Read the model definition and answer for the solid it produces. Units are mm, in the model's axes. A direction names the side the tool comes from. Give positions to 0.01 mm unless a question says otherwise; leave off trailing zeros. Write each loop counter-clockwise with the first axis right and the second up, starting at its lowest first coordinate (ties: lowest second). Pieces come first, ordered by that corner, then holes. Notation, with made-up numbers: M -15.5,-13.75 L 6.5,-13.75 A14 ccw 6.5,-3.75 Z; hole C 4,89 d8. An arc over 180 degrees is marked long. Use a Markdown table: item, result. Add a question column.
Item 1: Consider probe 1 along Y at (x, z) = (-22.5, -4.05); probe 2 along Y at (x, z) = (-52.5, -2.9); probe 3 along X at (y, z) = (-2, -3.85). Determine where each line is inside the solid, lowest interval first. Write a range as [from, to].
Item 2: A cutting plane is placed at A-A on z = -3.55. Determine the outline of the cut face in (x, y), then the cut area to 3 significant figures.
Item 3: The mould has two halves that part along X. Classify faces 1 (the flat face through (-36.032, -10.535, -2.958)), 2 (the flat face through (-38.34, 4.12, -2.96)), 3 (the flat face through (-37.19, -9.23, -2.96)): pulls with the +X half, pulls with the -X half, needs draft (parallel to the pull), parting line crosses it, or undercut.
Item 4: Given P1, Ø1, axis at x = -25.5, y = 4.5, coming from the +Z side; P2, Ø2, axis at y = -9.5, z = -2, coming from the -X side; P3, Ø1, axis at y = -6.5, z = -4.5, coming from the +X side; P4, Ø1, axis at y = -5.5, z = -1.5, coming from the -X side, each flat-ended and moving along its own axis, determine where each tip first touches the part or whether it passes through.
Item 5: A cutting plane is placed at C-C on x = -33.5. Determine the outline of the cut face in (y, z), then the cut area to 3 significant figures.
Item 6: For faces 4 (the flat face through (-37.183, 2.815, -2.958)), 5 (the flat face through (-37.4, -9.4, -6)), determine the directions among +Z, -Z, +X, -X, +Y, -Y from which every point of the face is accessible in a straight line to the end or side of a thin tool.
Item 7: A cutting plane is placed at B-B on y = 2.5. Determine the outline of the cut face in (x, z), then the cut area to 3 significant figures.
Autodesk Inventor part; units mm, degrees
ref_plane "YZ Plane" through (0, 0, 0) normal (1, 0, 0) x (0, 1, 0)
ref_plane "XZ Plane" through (0, 0, 0) normal (0, 1, 0) x (-1, 0, 0)
ref_plane "XY Plane" through (0, 0, 0) normal (0, 0, 1) x (1, 0, 0)
sketch "Эскиз1" plane through (0, 0, 0) normal (0, 0, 1) x (1, 0, 0)
  arc A0 (0.5156, -5.9778) -> (-0.5156, 5.9778) centre (0, 0) ccw
  arc A1 (0.6359, -7.3726) -> (-0.6359, 7.3726) centre (0, 0) ccw
  circle A2 centre (-74.3766, -6.4146) radius 2
  arc A3 (-74.8921, -0.4368) -> (-73.861, -12.3924) centre (-74.3766, -6.4146) ccw
  arc A4 (-75.0124, 0.9581) -> (-73.7407, -13.7872) centre (-74.3766, -6.4146) ccw
  line L0 (-75.0124, 0.9581) -> (-0.6359, 7.3726)
  line L1 (0.6359, -7.3726) -> (-73.7407, -13.7872)
  line L2 (-73.861, -12.3924) -> (0.5156, -5.9778)
  line L3 (-0.5156, 5.9778) -> (-74.8921, -0.4368)
  dimension "d0" = 12
  dimension "d1" = 1.4
  dimension "d2" = 12
  dimension "d3" = 1.4
extrude "Выдавливание1" add sketch "Эскиз1" against normal blind 6 contours L1 A4 L0 A1
properties part number "ремень оси y моторный"
Filled in:
| question | item | result |
|---|---|---|
| 1 | probe 1 | [-9.37, -7.96], [4.08, 5.49] |
| 1 | probe 2 | [-11.96, -10.55], [1.49, 2.9] |
| 1 | probe 3 | [-80.32, -78.44], [5.66, 7.12] |
| 2 | outline | M -75.01,0.96 A7.4 ccw -73.74,-13.79 L 0.64,-7.37 A7.4 ccw -0.64,7.37 Z; hole M -74.89,-0.44 A6 ccw -73.86,-12.39 L 0.52,-5.98 A6 ccw -0.52,5.98 Z |
| 2 | area | 268 mm² |
| 3 | face 1 | pulls with the +X half |
| 3 | face 2 | pulls with the -X half |
| 3 | face 3 | undercut |
| 4 | P1 | z = 0 |
| 4 | P2 | x = -81.48 |
| 4 | P3 | x = 4.33 |
| 4 | P4 | x = -81.77 |
| 5 | outline | M -10.32,-6 L -8.91,-6 L -8.91,0 L -10.32,0 Z; M 3.13,-6 L 4.54,-6 L 4.54,0 L 3.13,0 Z |
| 5 | area | 16.9 mm² |
| 6 | face 4 | +Z, -Z |
| 6 | face 5 | -Z, +X, -X, +Y, -Y |
| 7 | outline | M -57.13,-6 L -40.84,-6 L -40.84,0 L -57.13,0 Z; M 5.45,-6 L 6.96,-6 L 6.96,0 L 5.45,0 Z |
| 7 | area | 107 mm² |
